Could you check a few things on this model? Use its own coordinates, in mm. Give positions to 0.01 mm unless a question says otherwise; leave off trailing zeros. Order: outer loops, then holes, each group sorted by start corner. A loop starts at its lowest first (then second) coordinate and runs counter-clockwise, first axis right, second up. Notation, with made-up numbers: (88.5, -23) - (115.5, -23) arc R25 ccw to (115.5, 8) - close; hole circle Ø7 at (9.25, 87.25). An arc over 180 degrees is marked (long way). One line per question, with ' | ' between items. Start each with the question number.
1. I need wall thicknesses on probe 1 along Z at (x, y) = (-40, -20); probe 2 along Y at (x, z) = (-14, 26); probe 3 along X at (y, z) = (-29.5, 41). Which ranges of each line are inside material? Lowest first, please. Write a range as from..to.
2. Imagine slicing it at B-B (y = -23). Please give me the cut outline in (x, z).
3. For P1, Ø4, axis at x = -24.5, z = 30, coming from the +Y side; P2, Ø4, axis at x = -15, y = -52, coming from the +Z side; P3, Ø1.5, axis at x = -44.5, y = -15.5, coming from the +Z side; P4, Ø10, axis at x = -19, y = -34, coming from the -Z side, each with a flat end and sliding along its axis, tell me the tip position at first contact or that it passes through.
4. Imagine slicing it at A-A (x = -42.5). Please give me the cut outline in (y, z).
```python
from build123d import *

# Parameters (mm, degrees)
F0_W     = 76.2
F0_H     = 76.2
F1_DEPTH = 76.2
F4_DEPTH = 76.2
F5_DEPTH = 76.2


with BuildPart() as f1:
    # F0 (on Right) → F1 (new body)
    with BuildSketch(Plane.YZ):
        with Locations((-38.1, 38.1)):
            Rectangle(F0_W, F0_H)
    extrude(amount=-F1_DEPTH)

    # F3 (on face) → F4 (cut)
    with BuildSketch(Plane(origin=(-76.2, 0, 0), x_dir=(0, -1, 0), z_dir=(-1, 0, 0))):
        Polygon((0, 76.2), (0, 0), (38.1, 76.2), align=None)
        Polygon((38.1, 76.2), (76.2, 0), (76.2, 76.2), align=None)
    extrude(amount=-F4_DEPTH, mode=Mode.SUBTRACT)

    # F2 (on face) → F5 (cut)
    with BuildSketch(Plane.XZ.offset(76.2)):
        Polygon((-76.2, 0), (-38.1, 76.2), (-76.2, 76.2), align=None)
        Polygon((0, 76.2), (-38.1, 76.2), (0, 0), align=None)
    extrude(amount=-F5_DEPTH, mode=Mode.SUBTRACT)


solid = f1.part
```
Results found:
1) probe 1: z = 0..40 | probe 2: y = -63.2..-13 | probe 3: x = -55.7..-20.5
2) outline: (-76.2, 0) - (0, 0) - (-23, 46) - (-53.2, 46) - close
3) P1: stops at y = -14 | P2: stops at z = 34 | P3: stops at z = 32.5 | P4: stops at z = 0
4) outline: (-76.2, 0) - (0, 0) - (-33.7, 67.4) - (-42.5, 67.4) - close
